Check sheet for the modelled part. Datum: model origin and axes. Units: mm. Give positions to 0.01 mm unless a question says otherwise; leave off trailing zeros. Order: outer loops, then holes, each group sorted by start corner. A loop starts at its lowest first (then second) coordinate and runs counter-clockwise, first axis right, second up.
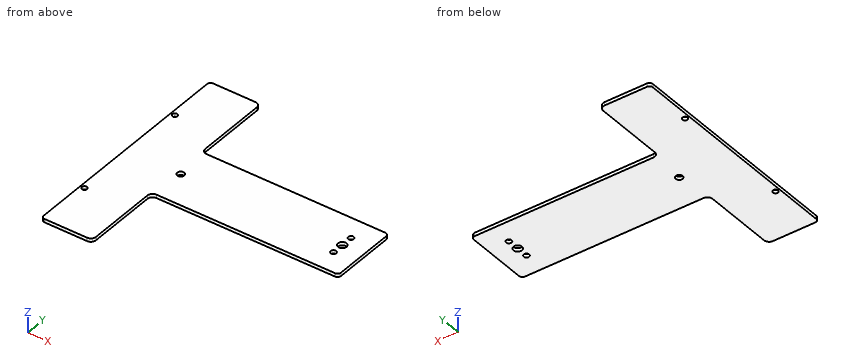
```python
from build123d import *

# Parameters (mm, degrees)
EXTRUDE_1_DEPTH     = 2
SKETCH_2_R          = 2.5
SKETCH_2_R_2        = 2
SKETCH_2_R_3        = 1.5
CUT_EXTRUDE_1_DEPTH = 2
SKETCH_3_R          = 1.6
CUT_EXTRUDE_2_DEPTH = 2


with BuildPart() as part:
    # 草图1 → 凸台-拉伸1 (new body)
    with BuildSketch(Plane.XY.offset(45.656070911)):
        with BuildLine():
            Line((82.078378746, 65), (82.078378746, -65))
            ThreePointArc((82.078378746, -65), (82.664165184, -66.414213562), (84.078378746, -67))
            Line((84.078378746, -67), (109, -67))
            ThreePointArc((109, -67), (111.121320344, -66.121320344), (112, -64))
            Line((112, -64), (112, -23))
            ThreePointArc((112, -23), (112.878679656, -20.878679656), (115, -20))
            Line((115, -20), (220.078378746, -20))
            ThreePointArc((220.078378746, -20), (221.492592308, -19.414213562), (222.078378746, -18))
            Line((222.078378746, -18), (222.078378746, 18))
            ThreePointArc((222.078378746, 18), (221.492592308, 19.414213562), (220.078378746, 20))
            Line((220.078378746, 20), (115, 20))
            ThreePointArc((115, 20), (112.878679656, 20.878679656), (112, 23))
            Line((112, 23), (112, 64))
            ThreePointArc((112, 64), (111.121320344, 66.121320344), (109, 67))
            Line((109, 67), (84.078378746, 67))
            ThreePointArc((84.078378746, 67), (82.664165184, 66.414213562), (82.078378746, 65))
        make_face()
    extrude(amount=EXTRUDE_1_DEPTH)

    # 草图2 → 切除-拉伸1 (cut)
    with BuildSketch(Plane.XY.offset(45.656070911)):
        with Locations((209.578378746, 0)):
            Circle(SKETCH_2_R)
        with Locations((114.578378746, 0)):
            Circle(SKETCH_2_R_2)
        with Locations((84.578378746, -36)):
            Circle(SKETCH_2_R_3)
        with Locations((84.578378746, 36)):
            Circle(SKETCH_2_R_3)
    extrude(amount=CUT_EXTRUDE_1_DEPTH, mode=Mode.SUBTRACT)

    # 草图3 → 切除-拉伸2 (cut)
    with BuildSketch(Plane.XY.offset(45.656070911)):
        with Locations((209.57858663, -7)):
            Circle(SKETCH_3_R)
        with Locations((209.57858663, 7)):
            Circle(SKETCH_3_R)
    extrude(amount=CUT_EXTRUDE_2_DEPTH, mode=Mode.SUBTRACT)


solid = part.part
```
(1) Thickness scan on L1, parallel to X at y = 46, z = 47.05; L2, parallel to Y at x = 192, z = 47.05; L3, parallel to X at y = -6, z = 46.15. Record the ranges inside material, lowest first.
(2) Go/stop test with flat-tipped pins: P1, Ø1, axis at y = -41, z = 46, coming from the +X side; P2, Ø1.8, axis at x = 84.58, y = -36, coming from the -Z side. Record where each tip stops, or that it passes through.
(3) Sectioned sample at A-A (y = -7). Enter the section's corners in (x, z), plus the area to 3 significant figures.
(4) Sectioned sample at B-B (z = 47.2). Enter the section's corners in (x, y).
(5) Sectioned sample at C-C (x = 205). Enter the section's corners in (y, z), plus the area to 3 significant figures.
(6) Sectioned sample at D-D (y = -44). Enter the section's corners in (x, z), plus the area to 3 significant figures.
Values follow:
1. L1: x = 82.08 to 112
1. L2: y = -20 to 20
1. L3: x = 82.08 to 208.33, 210.83 to 222.08
2. P1: stops at x = 112
2. P2: passes through
3. outline: (82.08, 45.66) - (207.98, 45.66) - (207.98, 47.66) - (82.08, 47.66) - close; (211.18, 45.66) - (222.08, 45.66) - (222.08, 47.66) - (211.18, 47.66) - close
3. area: 274 mm2
4. outline: (82.08, -65) arc R2 ccw to (84.08, -67) - (109, -67) arc R3 ccw to (112, -64) - (112, -23) arc R3 cw to (115, -20) - (220.08, -20) arc R2 ccw to (222.08, -18) - (222.08, 18) arc R2 ccw to (220.08, 20) - (115, 20) arc R3 cw to (112, 23) - (112, 64) arc R3 ccw to (109, 67) - (84.08, 67) arc R2 ccw to (82.08, 65) - close; hole circle Ø3 at (84.58, -36); hole circle Ø3 at (84.58, 36); hole circle Ø4 at (114.58, 0); hole circle Ø5 at (209.58, 0); hole circle Ø3.2 at (209.58, -7); hole circle Ø3.2 at (209.58, 7)
5. outline: (-20, 45.66) - (20, 45.66) - (20, 47.66) - (-20, 47.66) - close
5. area: 80.0 mm2
6. outline: (82.08, 45.66) - (112, 45.66) - (112, 47.66) - (82.08, 47.66) - close
6. area: 59.8 mm2
